Geometry check sheet. Reference: the model listing, model coordinates, mm. Give positions to 0.01 mm unless a question says otherwise; leave off trailing zeros. Loops run counter-clockwise (first coordinate to the right, second up) from the corner with the lowest first, then second, coordinate; pieces in that order, holes last. Notation, with made-up numbers: (-36.5, 42.5) - (-21.5, 42.5) arc R20 cw to (-21.5, 61.5) - close; hole circle Ø6 at (64, 14). An arc over 180 degrees is marked (long way). Use a Markdown table: item, result. Add a question column.
1. Material ranges on L1, parallel to Z at x = -40, y = -26, recorded low to high.
2. Depth check by flat-ended pin: P1, Ø2, axis at x = -12.5, y = 19, coming from the -Z side; P2, Ø1.5, axis at x = -24, z = -1.5, coming from the +Y side. Enter the tip coordinate at first touch or a pass-through.
3. Cross-section at C-C on y = 50. Enter the section's corners in (x, z), and give its area (3 significant figures).
4. Cross-section at A-A on z = -4. Count the separate pieces of the cut face and the enclosed holes in it, and give its area (3 significant figures).
5. Cross-section at B-B on x = 30. Enter the section's corners in (y, z), and give its area (3 significant figures).
from build123d import *

# Parameters (mm, degrees)
CROQUIS1_W              = 90
CROQUIS1_H              = 122
SALIENTE_EXTRUIR1_DEPTH = 15
CROQUIS2_R              = 0.8
SALIENTE_EXTRUIR2_DEPTH = 7


with BuildPart() as part:
    # Croquis1 → Saliente-Extruir1 (new body)
    with BuildSketch(Plane.XY):
        Rectangle(CROQUIS1_W, CROQUIS1_H)
    extrude(amount=SALIENTE_EXTRUIR1_DEPTH)

    # Croquis2 → Saliente-Extruir2 (add)
    with BuildSketch(Plane.XY):
        with Locations((10.16, -53.5)):
            Circle(CROQUIS2_R)
        with Locations((10.16, 53.5)):
            Circle(CROQUIS2_R)
        with Locations((5.08, -53.5)):
            Circle(CROQUIS2_R)
        with Locations((5.08, 53.5)):
            Circle(CROQUIS2_R)
        with Locations((0, -53.5)):
            Circle(CROQUIS2_R)
        with Locations((0, 53.5)):
            Circle(CROQUIS2_R)
        with Locations((-5.08, -53.5)):
            Circle(CROQUIS2_R)
        with Locations((-5.08, 53.5)):
            Circle(CROQUIS2_R)
        with Locations((-10.16, -53.5)):
            Circle(CROQUIS2_R)
        with Locations((-10.16, 53.5)):
            Circle(CROQUIS2_R)
    extrude(amount=-SALIENTE_EXTRUIR2_DEPTH)


solid = part.part
Values found:
| question | item | result |
|---|---|---|
| 1 | L1 | z = 0 to 15 |
| 2 | P1 | stops at z = 0 |
| 2 | P2 | passes through |
| 3 | outline | (-45, 0) - (45, 0) - (45, 15) - (-45, 15) - close |
| 3 | area | 1,350 mm2 |
| 4 | separate pieces | 10 |
| 4 | enclosed holes | 0 |
| 4 | area | 20.1 mm2 |
| 5 | outline | (-61, 0) - (61, 0) - (61, 15) - (-61, 15) - close |
| 5 | area | 1,830 mm2 |
